```python
from build123d import *

# Parameters (mm, degrees)
EXTRUDE_1_DEPTH = 10
SKETCH_2_R      = 20
EXTRUDE_2_DEPTH = 10


with BuildPart() as part:
    # 草图1 → 凸台-拉伸1 (new body)
    with BuildSketch(Plane.XY):
        with BuildLine():
            Line((-30, 0), (-30, -30))
            Line((-30, -30), (30, -30))
            Line((30, -30), (30, 0))
            ThreePointArc((30, 0), (0, 30), (-30, 0))
        make_face()
    extrude(amount=EXTRUDE_1_DEPTH)

    # 草图2 → 凸台-拉伸2 (add)
    with BuildSketch(Plane.XY.offset(10)):
        Circle(SKETCH_2_R)
    extrude(amount=EXTRUDE_2_DEPTH)


solid = part.part
```
Source: CAD feature listing. Evaluate the final solid. Frame: model axes, mm. A direction names the side the tool comes from. Coordinates: 2 decimals unless noted, no trailing zeros. Write each loop counter-clockwise with the first axis right and the second up, starting at its lowest first coordinate (ties: lowest second). Pieces come first, ordered by that corner, then holes. Notation, with made-up numbers: (-21, 29.25) -> (9, 29.25) arc R26 ccw to (9, 46.25) -> close; hole circle Ø9 at (25, 48). An arc over 180 degrees is marked (long way). Return JSON: item names as keys, results as strings. Group by question number.
1) Section query A-A, the plane x = 9.5. Return loops of the section in (y, z).
2) Section query B-B, the plane y = -15. Return loops of the section in (x, z).
3) Contact query for flat-ended pins moving along their axis: P1, Ø5, axis at x = -16.5, y = 23, coming from the -Z side; P2, Ø8, axis at x = 20, z = 17.5, coming from the -Y side. Output: stop coordinate, or through.
4) Ray query, line 1 along Z through (x, y) = (20, -17); line 2 along X through (y, z) = (-6, 10.25); line 3 along X through (y, z) = (-11, 17.75). Return the intervals inside material, ascending.
5) Section query D-D, the plane y = -22. Return loops of the section in (x, z), plus the area to 3 significant figures.
6) Section query C-C, the plane z = 6.5. Return loops of the section in (x, y).
7) Set-up query: faces 1 (the face through (0, 0, 0)), 2 (the face through (-4.336, -19.524, 14.93)). Return all of +Z, -Z, +X, -X, +Y, -Y with unobstructed straight access to the full face (end or side cutting, diameter ignored); none if empty.
From the geometry:
{
 "1": {"outline": "(-30, 0) -> (28.46, 0) -> (28.46, 10) -> (17.6, 10) -> (17.6, 20) -> (-17.6, 20) -> (-17.6, 10) -> (-30, 10) -> close"},
 "2": {"outline": "(-30, 0) -> (30, 0) -> (30, 10) -> (13.23, 10) -> (13.23, 20) -> (-13.23, 20) -> (-13.23, 10) -> (-30, 10) -> close"},
 "3": {"P1": "z = 0", "P2": "y = -12"},
 "4": {"line 1": "0 to 10", "line 2": "-19.08 to 19.08", "line 3": "-16.7 to 16.7"},
 "5": {"outline": "(-30, 0) -> (30, 0) -> (30, 10) -> (-30, 10) -> close", "area": "600 mm²"},
 "6": {"outline": "(-30, -30) -> (30, -30) -> (30, 0) arc R30 ccw to (-30, 0) -> close"},
 "7": {"face 1": "-Z, +X, -X, +Y, -Y", "face 2": "+Z"}
}
